Design review of the part shown in the three views and the two pictorial views. Dimensions are in mm from the part's minimum x, y and z. Round coordinates to 2 decimals unless told otherwise and drop trailing zeros. Loops run counter-clockwise (first coordinate to the right, second up) from the corner with the lowest first, then second, coordinate; pieces in that order, holes last. Notation, with made-up numbers: (-5.75, 79.25) -> (52.25, 79.25) arc R20 cw to (52.25, 93.25) -> close; hole circle Ø3 at (-27, 55.5). An arc over 180 degrees is marked (long way). Return JSON: item names as keys, results as strings. Group by question number.
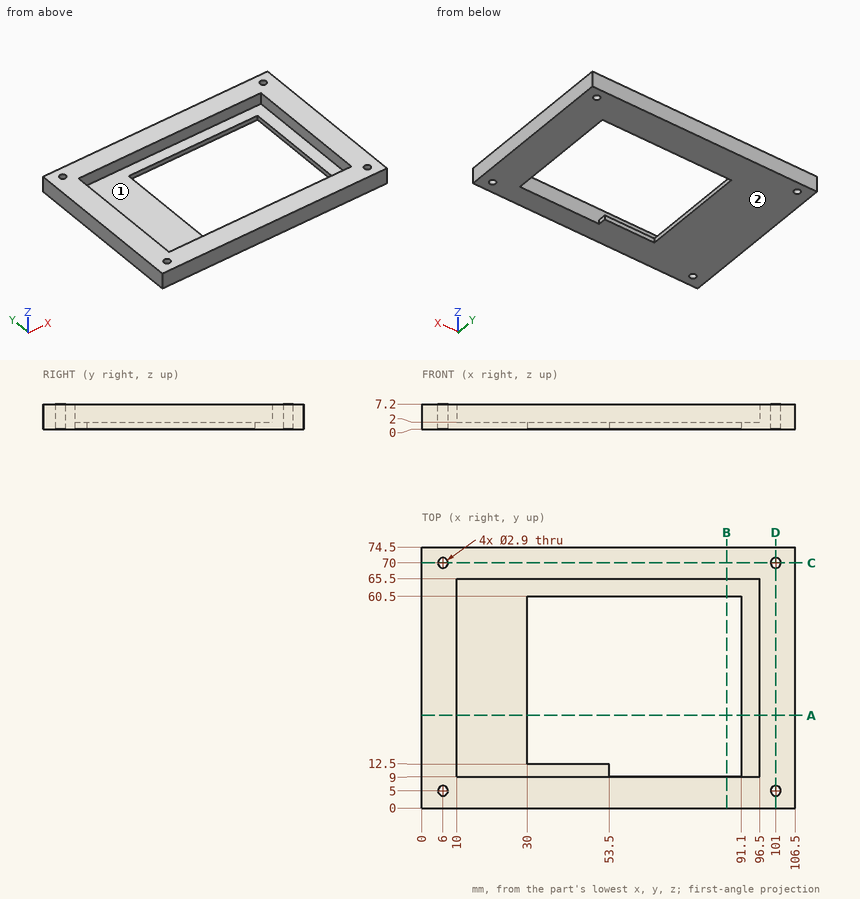
1. We need section A-A, the plane y = 26.5. Write out the cut boundary in (x, z), then the cut area to 3 significant figures.
2. For P1, Ø2.5, axis at x = 6, y = 70, coming from the -Z side; P2, Ø4, axis at x = 101, y = 5, coming from the -Z side, all flat-tipped, find the tip position at first contact; note any pin that passes through.
3. Draft analysis for pull direction Y (two halves, no side actions). For the marked faces 1 and 2, state which applies: pulls with the +Y half, pulls with the -Y half, needs draft (parallel to the pull), parting line crosses it, or undercut.
4. We need section B-B, the plane x = 87. Write out the cut boundary in (y, z), then the cut area to 3 significant figures.
5. We need section C-C, the plane y = 70. Write out the cut boundary in (x, z).
6. Wall thickness on line 1 (Y direction, x = 101, z = 3.25); line 2 (X direction, y = 5, z = 3); line 3 (Y direction, x = 86.5, z = 2.5): over which ranges is each line inside the solid? List them lowest first.
7. We need section D-D, the plane x = 101. Write out the cut boundary in (y, z), then the cut area to 3 significant figures.
Check sheet entries:
{
 "1": {"outline": "(0, 0) -> (30, 0) -> (30, 2) -> (10, 2) -> (10, 7.2) -> (0, 7.2) -> close; (91.1, 0) -> (106.5, 0) -> (106.5, 7.2) -> (96.5, 7.2) -> (96.5, 2) -> (91.1, 2) -> close", "area": "195 mm²"},
 "2": {"P1": "passes through", "P2": "stops at z = 0"},
 "3": {"face 1": "undercut", "face 2": "needs draft"},
 "4": {"outline": "(0, 0) -> (9, 0) -> (9, 7.2) -> (0, 7.2) -> close; (60.5, 0) -> (74.5, 0) -> (74.5, 7.2) -> (65.5, 7.2) -> (65.5, 2) -> (60.5, 2) -> close", "area": "140 mm²"},
 "5": {"outline": "(0, 0) -> (4.55, 0) -> (4.55, 7.2) -> (0, 7.2) -> close; (7.45, 0) -> (99.55, 0) -> (99.55, 7.2) -> (7.45, 7.2) -> close; (102.45, 0) -> (106.5, 0) -> (106.5, 7.2) -> (102.45, 7.2) -> close"},
 "6": {"line 1": "y = 0 to 3.55, 6.45 to 68.55, 71.45 to 74.5", "line 2": "x = 0 to 4.55, 7.45 to 99.55, 102.45 to 106.5", "line 3": "y = 0 to 9, 65.5 to 74.5"},
 "7": {"outline": "(0, 0) -> (3.55, 0) -> (3.55, 7.2) -> (0, 7.2) -> close; (6.45, 0) -> (68.55, 0) -> (68.55, 7.2) -> (6.45, 7.2) -> close; (71.45, 0) -> (74.5, 0) -> (74.5, 7.2) -> (71.45, 7.2) -> close", "area": "495 mm²"}
}
